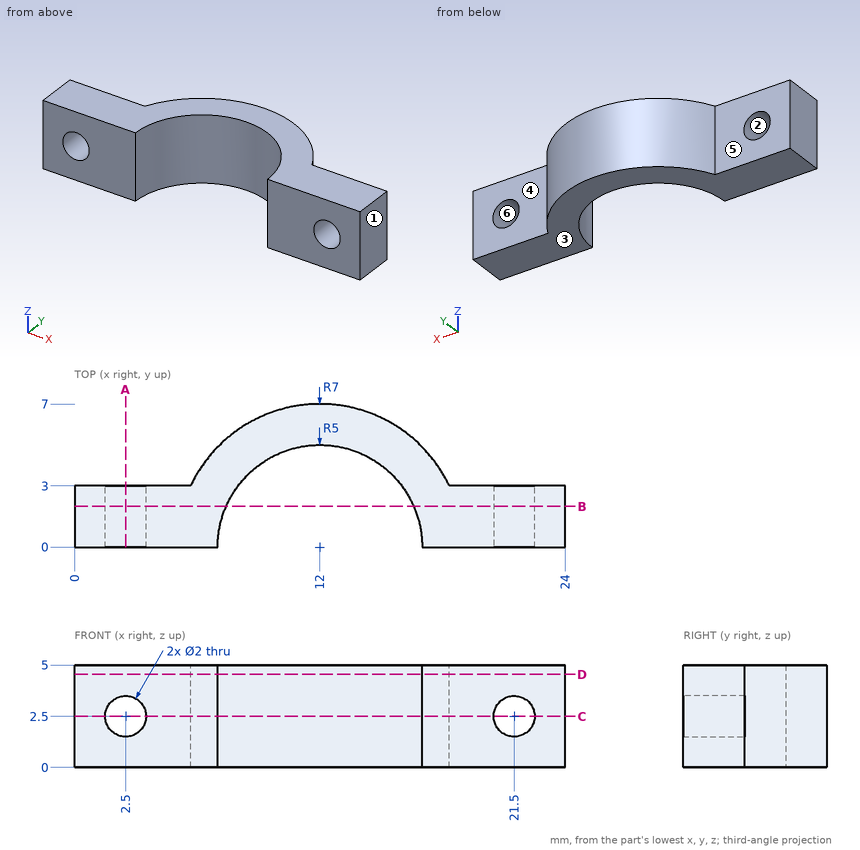
Print and shaded views of the part. All mm, measured from the part's lowest x, y and z. A direction names the side the tool comes from. Coordinates: 2 decimals unless noted, no trailing zeros. Write each loop counter-clockwise with the first axis right and the second up, starting at its lowest first coordinate (ties: lowest second). Pieces come first, ordered by that corner, then holes.
(1) Cut at C-C, the plane z = 2.5. List the corners of the cut face in (x, y), and give its area (3 significant figures).
(2) Drill centre lines: probe 1 along Z at (x, y) = (21.5, 1.55); probe 2 along X at (y, z) = (2.75, 3.2); probe 3 along Y at (x, z) = (19, 2.85). Where is each one in solid material? Low to high.
(3) Flat gauge pin, fed straight in: pin 1 (4 mm diameter, centred on x = 7.5, y = 5.5, fed in from +Z). Where does the tip first touch, or does it go through?
(4) Cut at D-D, the plane z = 4.55. List the corners of the cut face in (x, y), and give its area (3 significant figures).
(5) Cut at A-A, the plane x = 2.5. List the corners of the cut face in (y, z), and give its area (3 significant figures).
(6) Two-plate mould, pull along Z, no slides. Class the marked faces 1, 2 and 3: +Z half, -Z half, draft (parallel to the pull), parting line (faces both ways), or undercut.
(7) Cut at B-B, the plane y = 2. List the corners of the cut face in (x, z).
(8) 3-axis set-ups, long thin cutter, end or side, ignore diameter. For the marked faces 4, 5 and 6: which of +Z, -Z, +X, -X, +Y, -Y reach the whole face in a straight line?
Geometry says:
1. outline: (0, 0) - (1.5, 0) - (1.5, 3) - (0, 3) - close; (3.5, 0) - (7, 0) arc R5 cw to (17, 0) - (20.5, 0) - (20.5, 3) - (18.32, 3) arc R7 ccw to (5.68, 3) - (3.5, 3) - close; (22.5, 0) - (24, 0) - (24, 3) - (22.5, 3) - close
1. area: 57.0 mm2
2. probe 1: z = 0 to 1.5, 3.5 to 5
2. probe 2: x = 0 to 1.79, 3.21 to 7.82, 16.18 to 20.79, 22.21 to 24
2. probe 3: y = 0 to 3
3. pin 1: stops at z = 5
4. outline: (0, 0) - (7, 0) arc R5 cw to (17, 0) - (24, 0) - (24, 3) - (18.32, 3) arc R7 ccw to (5.68, 3) - (0, 3) - close
4. area: 69.0 mm2
5. outline: (0, 0) - (3, 0) - (3, 1.5) - (0, 1.5) - close; (0, 3.5) - (3, 3.5) - (3, 5) - (0, 5) - close
5. area: 9.00 mm2
6. face 1: draft
6. face 2: undercut
6. face 3: -Z half
7. outline: (0, 0) - (7.42, 0) - (7.42, 5) - (0, 5) - close; (16.58, 0) - (24, 0) - (24, 5) - (16.58, 5) - close; hole circle Ø2 at (2.5, 2.5); hole circle Ø2 at (21.5, 2.5)
8. face 4: +Z, -Z, +X, +Y
8. face 5: +Z, -Z, -X, +Y
8. face 6: +Y, -Y
